Autodesk Inventor part; units mm, degrees
ref_plane "Work Plane1" through (-30, 0, -23) normal (0, 0, 1) x (1, 0, 0)
ref_plane "YZ Plane" through (0, 0, 0) normal (1, 0, 0) x (0, 1, 0)
ref_plane "XZ Plane" through (0, 0, 0) normal (0, 1, 0) x (-1, 0, 0)
sketch "Sketch1" plane through (0, 0, 0) normal (0, 1, 0) x (-1, 0, 0)
  line L0 (0, 0) -> (30, 0)
  line L1 (30, 0) -> (30, -46)
  line L2 (30, -46) -> (0, -46)
  line L3 (0, -46) -> (0, 0)
  dimension "d0" = 30
  dimension "d1" = 46
extrude "Extrusion1" add sketch "Sketch1" along normal blind 6
sketch "Sketch2" plane through (-30, 0, 0) normal (0, 0, 1) x (1, 0, 0)
  line L0 (30, 0) -> (30, 6)
  line L1 (0, 0) -> (0, 6)
  point P0 (5, 3)
  point P1 (25, 3)
  point P2 (30, 3)
  point P3 (30, 3)
  dimension "d4" = 5
  dimension "d5" = 5
  dimension "d6" = 20
hole "Hole1" at (-25, 3, 0) at (-5, 3, 0) direction (0, 0, -1) diameter 2.459 depth 8.8 tip angle 118
ref_plane "Work Plane1" through (-30, 0, -23) normal (0, 0, 1) x (1, 0, 0)
mirror "Mirror1" about plane through (-30, 0, -23) normal (0, 0, 1) of "Hole1"
properties part number "Top_Separator Block" material "Aluminum 6061"
For this review, take the finished solid that the model builds, in its own axes (mm). A direction names the side the tool comes from. Coordinates: 2 decimals unless noted, no trailing zeros. Write each loop counter-clockwise with the first axis right and the second up, starting at its lowest first coordinate (ties: lowest second). Pieces come first, ordered by that corner, then holes. Notation, with made-up numbers: (52.25, 64.5) -> (73.25, 64.5) arc R13 ccw to (73.25, 78.5) -> close; hole circle Ø3 at (37.25, 9.5). An arc over 180 degrees is marked (long way). Put each result on its own line as item: value.
Q1. Tool access review of faces 4 (the flat face through (0, 3, -23)), 5 (the cylindrical face through (-6.09, 2.43, -41.54)), 6 (the cylindrical face through (-3.91, 2.43, -4.46)): name each direction out of +Z, -Z, +X, -X, +Y, -Y from which nothing blocks a thin tool from reaching the whole face with its end or side.
From the geometry:
face 4: +Z, -Z, +X, +Y, -Y
face 5: -Z
face 6: +Z
Q2. Take a section at A-A, the plane z = -40. State the section outline as (x, y) points, then the cut area to 3 significant figures.
From the geometry:
outline: (-30, 0) -> (0, 0) -> (0, 6) -> (-30, 6) -> close; hole circle Ø2.46 at (-25, 3); hole circle Ø2.46 at (-5, 3)
area: 171 mm2
Q3. The part is to be moulded in two halves that separate along Y. For faces 1 (the flat face through (-15, 0, -23)), 2 (the flat face through (-15, 3, -46)), 3 (the cylindrical face through (-26.2, 3.27, -41.54)), say which applies: +Y half, -Y half, draft (parallel to the pull), parting line (faces both ways), or undercut.
From the geometry:
face 1: -Y half
face 2: draft
face 3: undercut
Q4. Clearance check with flat-ended pins moving along their axes: pin 1 Ø2 at (x, y) = (-5, 3) entering from -Z; pin 2 Ø1.5 at (x, y) = (-25, 3) entering from +Z; pin 3 Ø2 at (x, y) = (-25, 3) entering from +Z. State where each tip first meets the part, or that it passes through.
From the geometry:
pin 1: stops at z = -37.06
pin 2: stops at z = -9.09
pin 3: stops at z = -8.94
Q5. Wall thickness on L1, parallel to Y at x = -5, z = -4.25; L2, parallel to X at y = 3, z = -40.5; L3, parallel to X at y = 3.65, z = -41: over which ranges is each line inside the solid? List them lowest first.
From the geometry:
L1: y = 0 to 1.77, 4.23 to 6
L2: x = -30 to -26.23, -23.77 to -6.23, -3.77 to 0
L3: x = -30 to -26.04, -23.96 to -6.04, -3.96 to 0
